Autodesk Inventor part; units mm, degrees
ref_plane "YZ Plane" through (0, 0, 0) normal (1, 0, 0) x (0, 1, 0)
ref_plane "XZ Plane" through (0, 0, 0) normal (0, 1, 0) x (-1, 0, 0)
ref_plane "XY Plane" through (0, 0, 0) normal (0, 0, 1) x (1, 0, 0)
sketch "Sketch1" plane through (0, 0, 0) normal (0, 1, 0) x (-1, 0, 0)
  line L0 (-152.4, 152.4) -> (152.4, 152.4)
  line L1 (152.4, 152.4) -> (152.4, -152.4)
  line L2 (152.4, -152.4) -> (-152.4, -152.4)
  line L3 (-152.4, -152.4) -> (-152.4, 152.4)
  line L4 (-152.4, 152.4) -> (152.4, -152.4) construction
  line L5 (152.4, 152.4) -> (-152.4, -152.4) construction
  point P0 (0, 0)
  dimension "d0" = 304.8
extrude "Extrusion1" add sketch "Sketch1" along normal blind 6.35
sketch "Sketch4" plane through (0, 6.35, 0) normal (0, 1, 0) x (1, 0, 0)
  line L0 (-152.4, -152.4) -> (152.4, -152.4) construction
  line L1 (152.4, -152.4) -> (152.4, 152.4) construction
  line L2 (152.4, 152.4) -> (-152.4, 152.4) construction
  line L3 (-152.4, 152.4) -> (-152.4, -152.4) construction
  line L4 (139.7, -139.7) -> (-139.7, -139.7) construction
  line L5 (-139.7, -139.7) -> (-139.7, 139.7) construction
  line L6 (-139.7, 139.7) -> (139.7, 139.7) construction
  line L7 (139.7, 139.7) -> (139.7, -139.7) construction
  line L8 (139.7, -139.7) -> (-139.7, 139.7) construction
  line L9 (-139.7, -139.7) -> (139.7, 139.7) construction
  point P0 (0, 0)
  point P1 (0, -139.7)
  point P2 (-139.7, 0)
  point P3 (0, 139.7)
  point P4 (139.7, 0)
  dimension "d21" = 279.4
  dimension "d22" = 279.4
hole "Hole2" at (-139.7, 6.35, 139.7) at (0, 6.35, 139.7) at (-139.7, 6.35, 0) at (-139.7, 6.35, -139.7) at (0, 6.35, -139.7) at (139.7, 6.35, -139.7) at (139.7, 6.35, 0) at (139.7, 6.35, 139.7) direction (0, -1, 0) diameter 6.528 depth 19.05 tip angle 118
sketch "Sketch2" plane through (0, 6.35, 0) normal (0, 1, 0) x (1, 0, 0)
  line L0 (-152.4, -152.4) -> (152.4, -152.4) construction
  line L1 (152.4, -152.4) -> (152.4, 152.4) construction
  line L2 (152.4, 152.4) -> (-152.4, 152.4) construction
  line L3 (-152.4, 152.4) -> (-152.4, -152.4) construction
  circle A0 centre (0, 0) radius 120.2565 construction
  line L4 (0, -152.4) -> (0, 152.4) construction
  line L5 (152.4, 152.4) -> (-152.4, 152.4) construction
  line L6 (-152.4, 0) -> (152.4, 0) construction
  point P0 (-120.2565, 0)
  point P1 (0, 120.2565)
  point P2 (120.2565, 0)
  point P3 (0, -120.2565)
  dimension "d3" = 240.513
hole "Hole1" at (-120.2565, 6.35, 0) at (0, 6.35, 120.2565) at (120.2565, 6.35, 0) at (0, 6.35, -120.2565) direction (0, -1, 0) diameter 4.978 depth 19.05 tip angle 118
sketch "Sketch3" plane through (0, 6.35, 0) normal (0, 1, 0) x (1, 0, 0)
  line L0 (-152.4, -152.4) -> (152.4, -152.4)
  line L1 (152.4, -152.4) -> (152.4, 152.4)
  line L2 (152.4, 152.4) -> (-152.4, 152.4)
  line L3 (-152.4, 152.4) -> (-152.4, -152.4)
  circle A0 centre (0, 0) radius 25
  dimension "d18" = 50
extrude "Extrusion3" cut sketch "Sketch3" against normal through all contours A0
properties part number "turntable-adapter-top" material "Acetal Resin, Black"
Geometry check sheet. Reference: the model listing, model coordinates, mm. Coordinates: 2 decimals unless noted, no trailing zeros. Order: outer loops, then holes, each group sorted by start corner. A loop starts at its lowest first (then second) coordinate and runs counter-clockwise, first axis right, second up.
Item 1: Section check B-B (y = 4). Count the separate pieces of the cut face and the enclosed holes in it, plus the area to 3 significant figures.
Item 2: Section check A-A (z = 7.5). Enter the section's corners in (x, y), plus the area to 3 significant figures.
Item 3: Depth check by flat-ended pin: pin 1 (10.5 mm diameter, centred on x = -139.7, z = -139.7, fed in from +Y). Enter the tip coordinate at first touch or a pass-through.
Item 4: Mould release check, pull along X, two halves, no side actions. Record for faces 1 (the flat face through (-32, 0, 2)), 2 (the cylindrical face through (-0.98, 3.131, -136.587)): released by +X, released by -X, zero draft, split by the parting line, or undercut.
Item 5: Scan lines: line 1 along Z through (x, y) = (-139.7, 1.5); line 2 along X through (y, z) = (3.75, 0). Record each from-to range of solid material in increasing order.
Check sheet entries:
1. separate pieces: 1
1. enclosed holes: 13
1. area: 90,600 mm2
2. outline: (-152.4, 0) - (-23.85, 0) - (-23.85, 6.35) - (-152.4, 6.35) - close; (23.85, 0) - (152.4, 0) - (152.4, 6.35) - (23.85, 6.35) - close
2. area: 1,630 mm2
3. pin 1: stops at y = 6.35
4. face 1: zero draft
4. face 2: undercut
5. line 1: z = -152.4 to -142.96, -136.44 to -3.26, 3.26 to 136.44, 142.96 to 152.4
5. line 2: x = -152.4 to -142.96, -136.44 to -122.75, -117.77 to -25, 25 to 117.77, 122.75 to 136.44, 142.96 to 152.4
